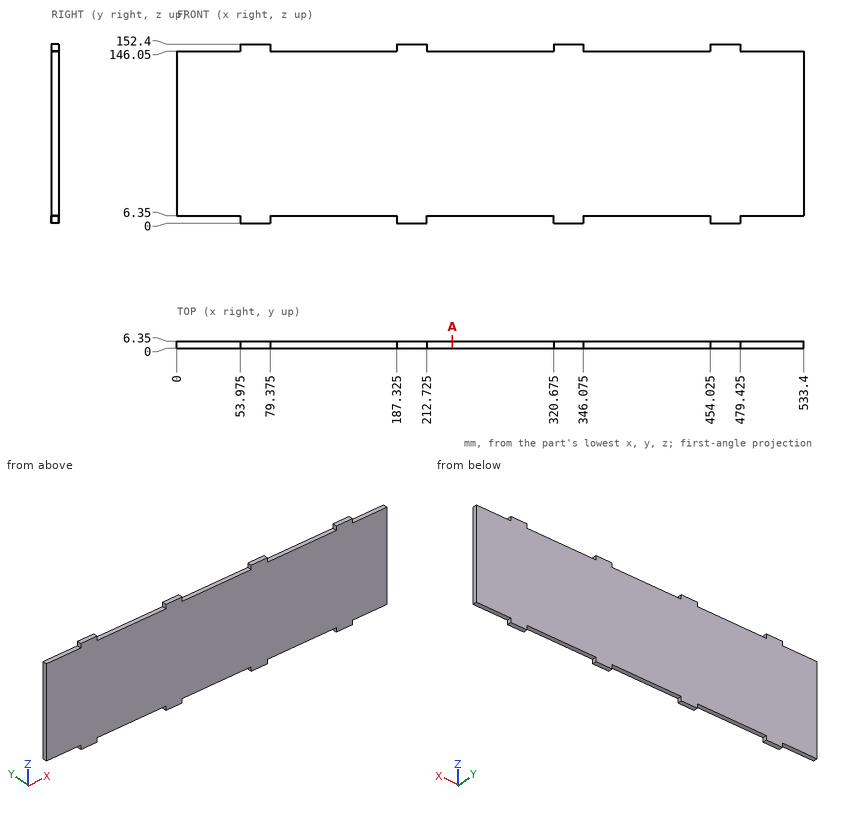
Here's the drawing with two shaded views (mm, measured from the low corner). I have some questions. Coordinates: 2 decimals unless noted, no trailing zeros. Order: outer loops, then holes, each group sorted by start corner. A loop starts at its lowest first (then second) coordinate and runs counter-clockwise, first axis right, second up.
Item 1: I need wall thicknesses on line 1 (Z direction, x = 167, y = 4). Which ranges of the line are inside material? Lowest first, please.
Result sheet:
line 1: z = 6.35 to 146.05
Item 2: For P1, Ø3, axis at y = 1.5, z = 148.5, coming from the -X side (3 decimals); P2, Ø1.9, axis at x = 507.5, y = 3.5, coming from the -Z side; P3, Ø3, axis at y = 4, z = 3, coming from the +X side (3 decimals), each with a flat end and sliding along its axis, tell me the tip position at first contact or that it passes through.
Result sheet:
P1: stops at x = 53.975
P2: stops at z = 6.35
P3: stops at x = 479.425
Item 3: If we section it at A-A on x = 234.5: List the corners of the cut face in (y, z) for me, plus the area to 3 significant figures.
Result sheet:
outline: (0, 6.35) - (6.35, 6.35) - (6.35, 146.05) - (0, 146.05) - close
area: 887 mm2
